Geometry check sheet. Reference: the model listing, model coordinates, mm. Face numbers are marked on the shaded views. A direction names the side the tool comes from. Give positions to 0.01 mm unless a question says otherwise; leave off trailing zeros. Order: outer loops, then holes, each group sorted by start corner. A loop starts at its lowest first (then second) coordinate and runs counter-clockwise, first axis right, second up. Notation, with made-up numbers: (26.25, 4) - (50.25, 4) arc R19 cw to (50.25, 36) - close; hole circle Ø2 at (-35.75, 17). An arc over 180 degrees is marked (long way). Put each result on its own line as item: value. Start each with the question number.
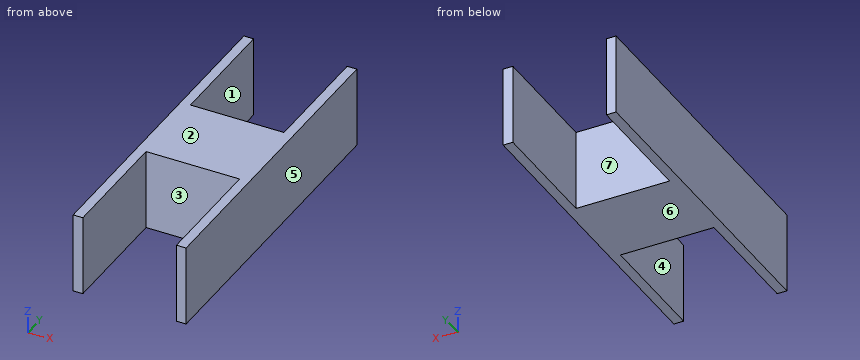
Autodesk Inventor part; units mm, degrees
ref_plane "YZ Plane" through (0, 0, 0) normal (1, 0, 0) x (0, 1, 0)
ref_plane "XZ Plane" through (0, 0, 0) normal (0, 1, 0) x (-1, 0, 0)
ref_plane "XY Plane" through (0, 0, 0) normal (0, 0, 1) x (1, 0, 0)
sketch "Sketch1" plane through (0, 0, 0) normal (0, 0, 1) x (1, 0, 0)
  line L0 (0, 80) -> (0, 0)
  line L1 (0, 0) -> (70, 0)
  line L2 (70, 0) -> (70, 80)
  line L3 (6, 80) -> (6, 6)
  line L4 (6, 6) -> (64, 6)
  line L5 (64, 6) -> (64, 80)
  line L6 (0, 80) -> (6, 80)
  line L7 (64, 80) -> (70, 80)
  line L8 (0, -20) -> (70, -20)
  line L9 (0, -120) -> (0, -40)
  line L10 (0, -40) -> (70, -40)
  line L11 (70, -40) -> (70, -120)
  line L12 (6, -120) -> (6, -46)
  line L13 (6, -46) -> (64, -46)
  line L14 (64, -46) -> (64, -120)
  line L15 (0, -120) -> (6, -120)
  line L16 (64, -120) -> (70, -120)
  dimension "d0" = 70
  dimension "d1" = 80
  dimension "d2" = 80
  dimension "d3" = 6
  dimension "d10" = 20
extrude "Extrusion1" add sketch "Sketch1" along normal blind 50
sketch "Sketch2" plane through (0, 0, 0) normal (0, -1, 0) x (1, 0, 0)
  line L0 (6, 0) -> (0, 0)
  line L1 (0, 50) -> (70, 50)
  line L2 (0, 0) -> (70, 0)
  line L3 (70, 0) -> (70, 50)
  line L4 (70, 50) -> (0, 50)
  line L5 (0, 50) -> (0, 0)
  line L6 (6, 6) -> (64, 6)
  line L7 (64, 6) -> (64, 44)
  line L8 (64, 44) -> (6, 44)
  line L9 (6, 44) -> (6, 6)
  dimension "d7" = 6
extrude "Extrusion2" add sketch "Sketch2" along normal blind 40
properties part number "armj3"
Item 1: Cross-section at A-A (y = 26). Enter the section's corners in (x, z).
Item 2: Cross-section at D-D (y = -35). Enter the section's corners in (x, z).
Item 3: Gauge pin test, flat ends, axial feed: pin 1 Ø2 at (x, z) = (47, 20) entering from -Y; pin 2 Ø11.5 at (x, z) = (29, 33.5) entering from +Y. Record the tip position at first contact, or that the pin passes through.
Item 4: Cross-section at C-C (x = 44.5). Enter the section's corners in (y, z).
Item 5: Thickness scan on line 1 along X through (y, z) = (-33.5, 29); line 2 along Z through (x, y) = (34.5, -15); line 3 along Y through (x, z) = (54, 32). Record the ranges inside material, lowest first.
Item 6: Release check for a two-part mould opening along X. For the marked faces 4, 5, 6 and 7 record: +X half, -X half, draft (parallel to the pull), parting line (faces both ways), or undercut.
Item 7: Set-up check for the marked faces 1, 2 and 3: record each of +Z, -Z, +X, -X, +Y, -Y from which the full face is reachable in a straight line by a thin tool's end or side.
Item 8: Cross-section at B-B (z = 41.5). Enter the section's corners in (x, y), and give its area (3 significant figures).
Recorded:
1. outline: (0, 0) - (6, 0) - (6, 50) - (0, 50) - close; (64, 0) - (70, 0) - (70, 50) - (64, 50) - close
2. outline: (0, 0) - (70, 0) - (70, 50) - (0, 50) - close; hole (6, 6) - (64, 6) - (64, 44) - (6, 44) - close
3. pin 1: stops at y = -46
3. pin 2: stops at y = 6
4. outline: (-46, 0) - (6, 0) - (6, 50) - (-46, 50) - close; hole (-40, 6) - (0, 6) - (0, 44) - (-40, 44) - close
5. line 1: x = 0 to 6, 64 to 70
5. line 2: z = 0 to 6, 44 to 50
5. line 3: y = -46 to -40, 0 to 6
6. face 4: undercut
6. face 5: +X half
6. face 6: draft
6. face 7: undercut
7. face 1: +Z, -Z, +Y
7. face 2: +Z, +X, -X, +Y, -Y
7. face 3: +Z, -Z, -Y
8. outline: (0, -120) - (6, -120) - (6, -46) - (64, -46) - (64, -120) - (70, -120) - (70, 80) - (64, 80) - (64, 6) - (6, 6) - (6, 80) - (0, 80) - close; hole (6, -40) - (64, -40) - (64, 0) - (6, 0) - close
8. area: 3,100 mm^2
